Geometry: final body of the model. Coordinates: model frame, mm. A direction names the side the tool comes from. Coordinates: 2 decimals unless noted, no trailing zeros. Write each loop counter-clockwise with the first axis right and the second up, starting at its lowest first coordinate (ties: lowest second). Pieces come first, ordered by that corner, then holes.
Autodesk Inventor part; units mm, degrees
ref_plane "YZ Plane" through (0, 0, 0) normal (1, 0, 0) x (0, 1, 0)
ref_plane "XZ Plane" through (0, 0, 0) normal (0, 1, 0) x (-1, 0, 0)
ref_plane "XY Plane" through (0, 0, 0) normal (0, 0, 1) x (1, 0, 0)
sketch "Sketch1" plane through (0, 0, 0) normal (1, 0, 0) x (0, 1, 0)
  line L0 (-10.2, -10.2) -> (10.2, -10.2)
  line L1 (10.2, -10.2) -> (10.2, 10.2)
  line L2 (10.2, 10.2) -> (-10.2, 10.2)
  line L3 (-10.2, 10.2) -> (-10.2, -10.2)
  line L4 (-10.2, -10.2) -> (10.2, 10.2) construction
  line L5 (10.2, -10.2) -> (-10.2, 10.2) construction
  point P0 (0, 0)
  dimension "d0" = 20.4
  dimension "d1" = 20.4
extrude "Extrusion1" add sketch "Sketch1" along normal blind 7.6
sketch "Sketch2" plane through (7.6, 0, 0) normal (1, 0, 0) x (0, 0, -1)
  circle A0 centre (0, 0) radius 12
  circle A1 centre (0, 0) radius 16.688
  dimension "d4" = 24
extrude "Extrusion2" cut sketch "Sketch2" against normal blind 7.6
sketch "Sketch3" plane through (7.6, 0, 0) normal (1, 0, 0) x (0, 0, -1)
  circle A0 centre (0, 0) radius 9.55
  dimension "d7" = 19.1
extrude "Extrusion3" add sketch "Sketch3" along normal blind 9.75
sketch "Sketch4" plane through (17.35, 0, 0) normal (1, 0, 0) x (0, 0, -1)
  circle A0 centre (0, 0) radius 8.05
  dimension "d10" = 16.1
extrude "Extrusion4" cut sketch "Sketch4" against normal blind 12.75
sketch "Sketch5" plane through (4.6, 0, 0) normal (1, 0, 0) x (0, 0, -1)
  point P0 (0, 0)
sketch "Sketch6" plane through (17.35, 0, 0) normal (1, 0, 0) x (0, 0, -1)
  point P0 (0, 0)
sketch "Sketch7" plane through (0, 0, 0) normal (-1, 0, 0) x (0, 0, 1)
  circle A0 centre (0, 0) radius 3.175
  dimension "d13" = 6.35
extrude "Extrusion5" cut sketch "Sketch7" against normal blind 12.75
sketch "Sketch8" plane through (0, 0, 0) normal (-1, 0, 0) x (0, 0, 1)
  point P0 (0, 0)
properties part number "thiccBB_hubs"
Item 1: Pin query (flat end, axial travel): pin 1 (1 mm diameter, centred on x = 15, y = 1, fed in from -Z); pin 2 (1.5 mm diameter, centred on y = -6.5, z = 2.5, fed in from +X); pin 3 (1.5 mm diameter, centred on x = 8, y = 7, fed in from -Z). Return the tip coordinate at first contact, or that it passes through.
Derived:
pin 1: stops at z = -9.54
pin 2: stops at x = 4.6
pin 3: stops at z = -10.17
Item 2: Set-up query: faces 1 (the cylindrical face through (12.41, 5.81, 7.58)), 2 (the flat face through (0, -2.4, 2.4)). Return all of +Z, -Z, +X, -X, +Y, -Y with unobstructed straight access to the full face (end or side cutting, diameter ignored); none if empty.
Derived:
face 1: +X
face 2: +Z, -Z, -X, +Y, -Y
Item 3: Material intervals for probe 1 along Y at (x, z) = (11.5, 0); probe 2 along X at (y, z) = (-7.5, 9); probe 3 along X at (y, z) = (-6, 3.25), sorted ascending.
Derived:
probe 1: y = -9.55 to -8.05, 8.05 to 9.55
probe 2: x = 0 to 7.6
probe 3: x = 0 to 4.6
Item 4: Section B-B, the plane x = 7. Output: boundary loops of the cut face in (y, z).
Derived:
outline: (-10.2, -6.32) arc R12 ccw to (-6.32, -10.2) - (6.32, -10.2) arc R12 ccw to (10.2, -6.32) - (10.2, 6.32) arc R12 ccw to (6.32, 10.2) - (-6.32, 10.2) arc R12 ccw to (-10.2, 6.32) - close; hole circle Ø16.1 at (0, 0)
Item 5: Pull-direction query (Y, two-part tool) for faces 3 (the flat face through (7.6, -7, 7)), 4 (the flat face through (4.6, 0.1, -3.5)), 5 (the cylindrical face through (3.85, 8.46, -8.51)); classes: released by +Y, released by -Y, zero draft, split by the parting line, or undercut.
Derived:
face 3: zero draft
face 4: undercut
face 5: released by +Y
Item 6: Section D-D, the plane y = -5.75. Output: boundary loops of the cut face in (x, z), plus the area to 3 significant figures.
Derived:
outline: (0, -10.2) - (7.6, -10.2) - (7.6, -7.62) - (17.35, -7.62) - (17.35, -5.63) - (4.6, -5.63) - (4.6, 5.63) - (17.35, 5.63) - (17.35, 7.62) - (7.6, 7.62) - (7.6, 10.2) - (0, 10.2) - close
area: 160 mm2
Item 7: Section A-A, the plane y = 0. Output: boundary loops of the cut face in (x, z) (3 decimals), plus the area to 3 significant figures.
Derived:
outline: (0, -10.2) - (7.6, -10.2) - (7.6, -9.55) - (17.35, -9.55) - (17.35, -8.05) - (4.6, -8.05) - (4.6, -3.175) - (0, -3.175) - close; (0, 3.175) - (4.6, 3.175) - (4.6, 8.05) - (17.35, 8.05) - (17.35, 9.55) - (7.6, 9.55) - (7.6, 10.2) - (0, 10.2) - close
area: 107 mm2
